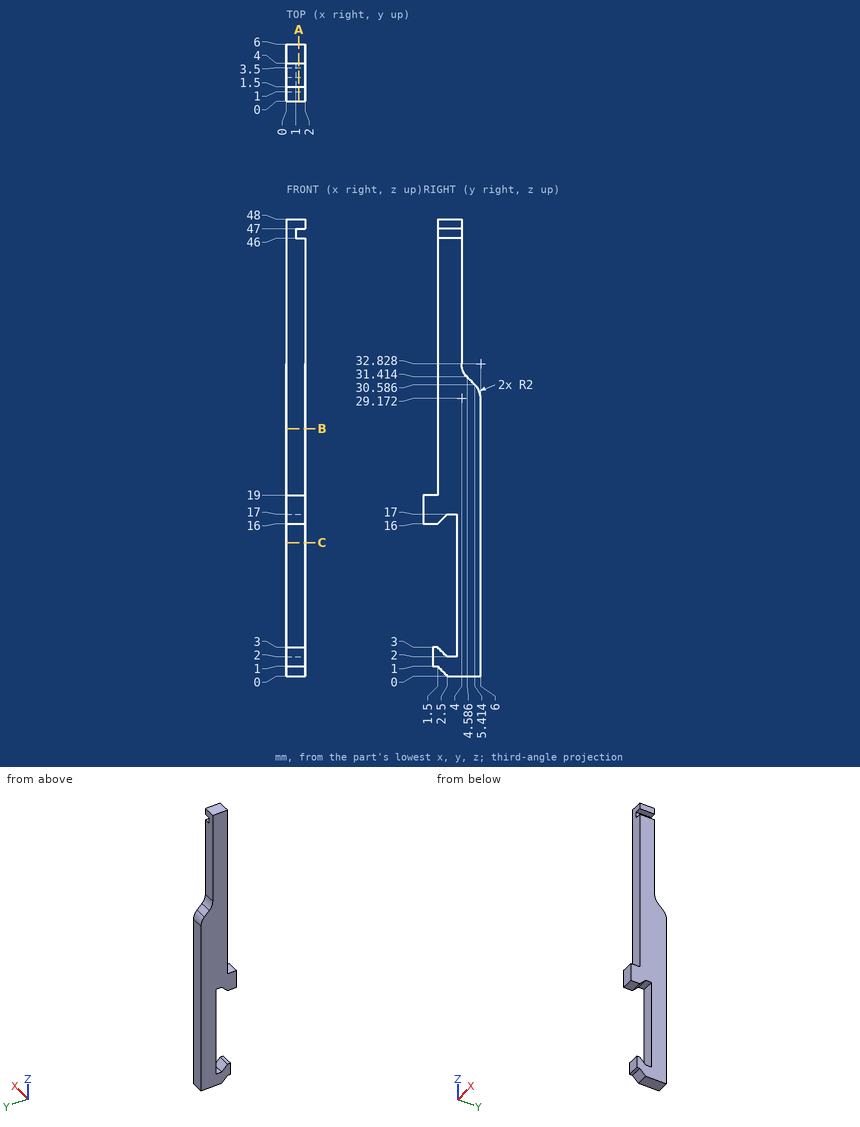
Part print with two shaded views. Sizes in mm from the minimum x, y, z corner. Round coordinates to 2 decimals unless told otherwise and drop trailing zeros. Order: outer loops, then holes, each group sorted by start corner. A loop starts at its lowest first (then second) coordinate and runs counter-clockwise, first axis right, second up.
(1) Band-saw the part on C-C (z = 14). List the corners of the cut face in (x, y).
(2) Band-saw the part on A-A (x = 1.3). List the corners of the cut face in (y, z) (1 decimal).
(3) Band-saw the part on B-B (z = 26). List the corners of the cut face in (x, y).
(4) Pin check, flat tips, straight feed: pin 1 (1 mm diameter, centred on x = 0.5, y = 1.5, fed in from -Z); pin 2 (0.5 mm diameter, centred on y = 2.5, z = 46.5, fed in from +X); pin 3 (1 mm diameter, centred on x = 1.5, z = 2.5, fed in from -Y). Stop position of each tip, or through.
(5) Drill centre lines: line 1 (Z direction, x = 1.75, y = 3.15); line 2 (Z direction, x = 0.7, y = 2.7); line 3 (Z direction, x = 0.9, y = 0.35). Where is each one in solid material? Low to high.
Verdict:
1. outline: (0, 3.5) - (2, 3.5) - (2, 6) - (0, 6) - close
2. outline: (0, 16) - (1.5, 16) - (2.5, 17) - (3.5, 17) - (3.5, 2) - (2.5, 2) - (1.5, 3) - (1, 3) - (1, 1) - (1.5, 1) - (2.5, 0) - (6, 0) - (6, 29.2) arc R2 ccw to (5.4, 30.6) - (4.6, 31.4) arc R2 cw to (4, 32.8) - (4, 46) - (1.5, 46) - (1.5, 19) - (0, 19) - close; (1.5, 47) - (4, 47) - (4, 48) - (1.5, 48) - close
3. outline: (0, 1.5) - (2, 1.5) - (2, 6) - (0, 6) - close
4. pin 1: stops at z = 0.5
4. pin 2: stops at x = 1
4. pin 3: stops at y = 1
5. line 1: z = 0 to 2, 17 to 46, 47 to 48
5. line 2: z = 0 to 2, 17 to 48
5. line 3: z = 16 to 19
